```python
from build123d import *

# Parameters (mm, degrees)
F0_W     = 15.77
F0_H     = 7.75
F1_DEPTH = 3.16
F2_R     = 2.45
F3_DEPTH = 1.99
F4_T     = -1.55
F5_R     = 1.2096188734
F5_R_2   = 0.9825120615
F6_DEPTH = 2


with BuildPart() as f1:
    # F0 (on Front) → F1 (new body)
    with BuildSketch(Plane.XZ):
        with Locations((-7.885, 3.875)):
            Rectangle(F0_W, F0_H)
    extrude(amount=F1_DEPTH)

    # F2 (on face) → F3 (join)
    with BuildSketch(Plane.XZ.offset(3.16)):
        with Locations((-12.5210902126, 3.7908264088)):
            Circle(F2_R)
        with Locations((-3.25, 3.8467605594)):
            Circle(F2_R)
    extrude(amount=F3_DEPTH)

    # F4
    f4_openings = [f1.faces().sort_by_distance(p)[0] for p in [
        (-7.885, 0, 3.875),
    ]]
    offset(amount=F4_T, openings=f4_openings, kind=Kind.INTERSECTION)

    # F5 (on Front) → F6 (join)
    with BuildSketch(Plane.XZ):
        with Locations((-7.8559592366, 3.8379097823)):
            Circle(F5_R)
        with Locations((-7.8559592366, 3.8379097823)):
            Circle(F5_R_2, mode=Mode.SUBTRACT)
    extrude(amount=F6_DEPTH)


solid = f1.part
```
For this review, take the finished solid that the model builds, in its own axes (mm). A direction names the side the tool comes from. Round coordinates to 2 decimals unless told otherwise and drop trailing zeros. Write each loop counter-clockwise with the first axis right and the second up, starting at its lowest first coordinate (ties: lowest second). Pieces come first, ordered by that corner, then holes. Notation, with made-up numbers: (-24, 53.25) -> (3, 53.25) arc R24 ccw to (3, 88.25) -> close; hole circle Ø2 at (59, -1). An arc over 180 degrees is marked (long way). One line per question, with ' | ' between items. Start each with the question number.
1) Mouldability with a two-part tool opening along X and no side actions: class faces 1 (the flat face through (-15.77, -2, 4)), 2 (the flat face through (0, -2, 4)), 3 (the flat face through (-8, -3.16, 4)) as +X half, -X half, draft (parallel to the pull), parting line (faces both ways), or undercut.
2) Wall thickness on line 1 along Z through (x, y) = (-3.25, -2.1); line 2 along Z through (x, y) = (-2.25, -1.1); line 3 along X through (y, z) = (-0.65, 4.25): over which ranges is each line inside the solid? List them lowest first.
3) For pin 1 Ø2 at (x, z) = (-3.5, 4) entering from +Y; pin 2 Ø3.5 at (x, z) = (-10, 4.5) entering from +Y; pin 3 Ø1.2 at (x, z) = (-7.86, 3.84) entering from -Y, all flat-tipped, find the tip position at first contact; note any pin that passes through.
4) Add section B-B (x = -3.25). Write out the cut boundary in (y, z), and give its area (3 significant figures).
5) Add section D-D (z = 5.5). Write out the cut boundary in (x, y).
6) Add section A-A (y = -1.3). Write out the cut boundary in (x, z).
7) Add section C-C (y = -4.75). Write out the cut boundary in (x, z), and give its area (3 significant figures).
8) Machinability: for faces 4 (the flat face through (-9.4, -1.61, 3.9)), 5 (the flat face through (-8, -2, 7.75)), 6 (the cylindrical face through (-10.184, -4.141, 4.527)), which of the approach directions +Z, -Z, +X, -X, +Y, -Y give a long, thin tool a straight path to every point of the face, cutting with its end or side? Answer none if there is none.
Reported:
1) face 1: -X half | face 2: +X half | face 3: undercut
2) line 1: z = 0 to 2.95, 4.75 to 7.75 | line 2: z = 0 to 1.55, 6.2 to 7.75 | line 3: x = -15.77 to -14.22, -8.99 to -8.75, -6.96 to -6.72, -1.55 to 0
3) pin 1: stops at y = -1.61 | pin 2: stops at y = 0 | pin 3: stops at y = -3.16
4) outline: (-5.15, 1.4) -> (-3.16, 1.4) -> (-3.16, 0) -> (0, 0) -> (0, 1.55) -> (-1.61, 1.55) -> (-1.61, 2.95) -> (-3.6, 2.95) -> (-3.6, 4.75) -> (-1.61, 4.75) -> (-1.61, 6.2) -> (0, 6.2) -> (0, 7.75) -> (-3.16, 7.75) -> (-3.16, 6.3) -> (-5.15, 6.3) -> close | area: 23.2 mm²
5) outline: (-15.77, -3.16) -> (-14.28, -3.16) -> (-14.28, -5.15) -> (-10.77, -5.15) -> (-10.77, -3.16) -> (-5.06, -3.16) -> (-5.06, -5.15) -> (-1.44, -5.15) -> (-1.44, -3.16) -> (0, -3.16) -> (0, 0) -> (-1.55, 0) -> (-1.55, -1.61) -> (-14.22, -1.61) -> (-14.22, 0) -> (-15.77, 0) -> close
6) outline: (-15.77, 0) -> (0, 0) -> (0, 7.75) -> (-15.77, 7.75) -> close; circle Ø2.42 at (-7.86, 3.84); hole (-14.22, 1.55) -> (-1.55, 1.55) -> (-1.55, 6.2) -> (-14.22, 6.2) -> close; hole circle Ø1.97 at (-7.86, 3.84)
7) outline: circle Ø4.9 at (-12.52, 3.79); circle Ø4.9 at (-3.25, 3.85) | area: 37.7 mm²
8) face 4: +Y | face 5: +Z, +X, -X, +Y, -Y | face 6: -Y
